```python
from build123d import *

# Parameters (mm, degrees)
SKETCH1_W           = 30.5
SKETCH1_H           = 34
BOSS_EXTRUDE1_DEPTH = 1.5
BOSS_EXTRUDE2_DEPTH = 3
SKETCH3_W           = 3
SKETCH3_H           = 8
SKETCH3_W_2         = 8
SKETCH3_H_2         = 3
BOSS_EXTRUDE3_DEPTH = 3
CUT_EXTRUDE1_DEPTH  = 4.0000001
CUT_EXTRUDE2_DEPTH  = 4.0000001
SKETCH6_W           = 8
SKETCH6_H           = 3
CUT_EXTRUDE3_DEPTH  = 4.0000001
CUT_EXTRUDE4_DEPTH  = 4.0000001
CUT_EXTRUDE6_DEPTH  = 4.0000001
SKETCH9_W           = 3
SKETCH9_H           = 4
BOSS_EXTRUDE4_DEPTH = 3
CUT_EXTRUDE7_DEPTH  = 4
FILLET1_R           = 3
BOSS_EXTRUDE5_DEPTH = 3


with BuildPart() as part:
    # Sketch1 → Boss-Extrude1 (new body, symmetric)
    with BuildSketch(Plane(origin=(0, 0, 0), x_dir=(1, 0, 0), z_dir=(0, 1, 0))):
        Rectangle(SKETCH1_W, SKETCH1_H)
    extrude(amount=BOSS_EXTRUDE1_DEPTH, both=True)

    # Sketch2 → Boss-Extrude2 (add)
    with BuildSketch(Plane(origin=(0, 1.5, 0), x_dir=(1, 0, 0), z_dir=(0, 1, 0))):
        with BuildLine():
            Line((-15.25, 17), (-24.07, 1.308996208))
            add(Edge.make_bspline(
                [(-24.07, 1.308996208), (-25.612124036, -1.43448158), (-30.226003395, -1.5229993), (-46.69780929, -11.088418218), (-55.382760657, -10.307171359), (-55.382760657, -17)],
                knots=[0, 0, 0, 0, 0.221130071, 0.603599568, 1, 1, 1, 1], degree=3))
            Line((-55.382760657, -17), (-15.25, -17))
            Line((-15.25, -17), (-15.25, 17))
        make_face()
    extrude(amount=-BOSS_EXTRUDE2_DEPTH)

    # Sketch3 → Boss-Extrude3 (add)
    with BuildSketch(Plane(origin=(0, 1.5, 0), x_dir=(1, 0, 0), z_dir=(0, 1, 0))):
        with Locations((16.75, 10)):
            Rectangle(SKETCH3_W, SKETCH3_H)
        with Locations((16.75, -10)):
            Rectangle(SKETCH3_W, SKETCH3_H)
        with Locations((-11.25, 18.5)):
            Rectangle(SKETCH3_W_2, SKETCH3_H_2)
        with Locations((11.25, 18.5)):
            Rectangle(SKETCH3_W_2, SKETCH3_H_2)
        with Locations((-51.382760657, -18.5)):
            Rectangle(SKETCH3_W_2, SKETCH3_H_2)
        with Locations((11.25, -18.5)):
            Rectangle(SKETCH3_W_2, SKETCH3_H_2)
        with Locations((-20.066380328, -18.5)):
            Rectangle(SKETCH3_W_2, SKETCH3_H_2)
    extrude(amount=-BOSS_EXTRUDE3_DEPTH)

    # Sketch4 → Cut-Extrude1 (cut, through all)
    with BuildSketch(Plane(origin=(0, 1.5, 0), x_dir=(1, 0, 0), z_dir=(0, 1, 0))):
        Polygon((-2.008190164, -14), (-2.008190164, -12.2), (-3.258190164, -12.2), (-3.258190164, -10), (-5.558190164, -10), (-5.558190164, -12.2), (-6.808190164, -12.2), (-6.808190164, -14), (-5.558190164, -14), (-5.558190164, -17), (-3.258190164, -17), (-3.258190164, -14), align=None)
        Polygon((-33.324570493, -14), (-33.324570493, -12.2), (-34.574570493, -12.2), (-34.574570493, -10), (-36.874570493, -10), (-36.874570493, -12.2), (-38.124570493, -12.2), (-38.124570493, -14), (-36.874570493, -14), (-36.874570493, -17), (-34.574570493, -17), (-34.574570493, -14), align=None)
    extrude(amount=-CUT_EXTRUDE1_DEPTH, mode=Mode.SUBTRACT)

    # Sketch5 → Cut-Extrude2 (cut, through all)
    with BuildSketch(Plane(origin=(0, 1.5, 0), x_dir=(1, 0, 0), z_dir=(0, 1, 0))):
        with BuildLine():
            Line((10.75, 20), (10.75, 7.75))
            ThreePointArc((10.75, 7.75), (2.5, -0.5), (-5.75, 7.75))
            Line((-5.75, 7.75), (-5.75, 20))
            Line((-5.75, 20), (10.75, 20))
        make_face()
    extrude(amount=-CUT_EXTRUDE2_DEPTH, mode=Mode.SUBTRACT)

    # Sketch6 → Cut-Extrude3 (cut, through all)
    with BuildSketch(Plane(origin=(0, 1.5, 0), x_dir=(1, 0, 0), z_dir=(0, 1, 0))):
        with Locations((-11.25, 18.5)):
            Rectangle(SKETCH6_W, SKETCH6_H)
    extrude(amount=-CUT_EXTRUDE3_DEPTH, mode=Mode.SUBTRACT)

    # Sketch7 → Cut-Extrude4 (cut, through all)
    with BuildSketch(Plane(origin=(0, 1.5, 0), x_dir=(1, 0, 0), z_dir=(0, 1, 0))):
        Polygon((-11.65, 17), (-9.35, 17), (-9.35, 14), (-8.1, 14), (-8.1, 12.2), (-9.35, 12.2), (-9.35, 10), (-11.65, 10), (-11.65, 12.2), (-12.9, 12.2), (-12.9, 14), (-11.65, 14), align=None)
    extrude(amount=-CUT_EXTRUDE4_DEPTH, mode=Mode.SUBTRACT)

    # Sketch8 → Cut-Extrude6 (cut, through all)
    with BuildSketch(Plane(origin=(0, 1.5, 0), x_dir=(1, 0, 0), z_dir=(0, 1, 0))):
        with BuildLine():
            Line((-24.066380328, -17), (-24.066380328, 1.315435696))
            Line((-24.066380328, 1.315435696), (-24.07, 1.308996208))
            add(Edge.make_bspline(
                [(-24.07, 1.308996208), (-25.612124036, -1.43448158), (-30.226003395, -1.5229993), (-46.69780929, -11.088418218), (-55.382760657, -10.307171359), (-55.382760657, -17)],
                knots=[0, 0, 0, 0, 0.221130071, 0.603599568, 1, 1, 1, 1], degree=3))
            Line((-55.382760657, -17), (-55.382760657, -20))
            Line((-55.382760657, -20), (-47.382760657, -20))
            Line((-47.382760657, -20), (-47.382760657, -17))
            Line((-47.382760657, -17), (-36.874570493, -17))
            Line((-36.874570493, -17), (-36.874570493, -14))
            Line((-36.874570493, -14), (-38.124570493, -14))
            Line((-38.124570493, -14), (-38.124570493, -12.2))
            Line((-38.124570493, -12.2), (-36.874570493, -12.2))
            Line((-36.874570493, -12.2), (-36.874570493, -10))
            Line((-36.874570493, -10), (-34.574570493, -10))
            Line((-34.574570493, -10), (-34.574570493, -12.2))
            Line((-34.574570493, -12.2), (-33.324570493, -12.2))
            Line((-33.324570493, -12.2), (-33.324570493, -14))
            Line((-33.324570493, -14), (-34.574570493, -14))
            Line((-34.574570493, -14), (-34.574570493, -17))
            Line((-34.574570493, -17), (-24.066380328, -17))
        make_face()
    extrude(amount=-CUT_EXTRUDE6_DEPTH, mode=Mode.SUBTRACT)

    # Sketch9 → Boss-Extrude4 (add)
    with BuildSketch(Plane(origin=(0, 1.5, 0), x_dir=(1, 0, 0), z_dir=(0, 1, 0))):
        with Locations((-25.566380328, -11)):
            Rectangle(SKETCH9_W, SKETCH9_H)
    extrude(amount=-BOSS_EXTRUDE4_DEPTH)

    # Sketch10 → Cut-Extrude7 (cut, through all)
    with BuildSketch(Plane(origin=(0, 1.5, 0), x_dir=(1, 0, 0), z_dir=(0, 1, 0))):
        with BuildLine():
            Line((-21.066380328, 0.530062836), (-21.066380328, -14.173024042))
            Line((-21.066380328, -14.173024042), (-9.808190164, -14.173024042))
            Line((-9.808190164, -14.173024042), (-9.808190164, -7))
            Line((-9.808190164, -7), (0.991809836, -7))
            Line((0.991809836, -7), (0.991809836, -14.173024042))
            Line((0.991809836, -14.173024042), (12.25, -14.173024042))
            Line((12.25, -14.173024042), (12.25, 2.13751392))
            ThreePointArc((12.25, 2.13751392), (-0.04063544, -3.20936456), (-8.72497216, 7))
            Line((-8.72497216, 7), (-17.429592871, 7))
            Line((-17.429592871, 7), (-21.066380328, 0.530062836))
        make_face()
    extrude(amount=-CUT_EXTRUDE7_DEPTH, mode=Mode.SUBTRACT)

    # Fillet1
    fillet1_edges = [part.edges().sort_by_distance(p)[0] for p in [
        (-21.066380328, 0, -0.530062836),
        (-17.429592871, 0, -7),
        (-8.72497216, 0, -7),
        (12.25, 0, -2.13751392),
        (12.25, 0, 14.173024042),
        (0.991809836, 0, 14.173024042),
        (-9.808190164, 0, 7),
        (-9.808190164, 0, 14.173024042),
        (-21.066380328, 0, 14.173024042),
    ]]
    fillet(fillet1_edges, radius=FILLET1_R)

    # Sketch11 → Boss-Extrude5 (add)
    with BuildSketch(Plane(origin=(0, 1.5, 0), x_dir=(1, 0, 0), z_dir=(0, 1, 0))):
        with BuildLine():
            Line((-4.256338517, -7), (0.991809836, -7))
            ThreePointArc((0.991809836, -7), (1.882552513, -4.608606487), (4.120680317, -3.382649968))
            ThreePointArc((4.120680317, -3.382649968), (0.464289311, -3.31428407), (-2.97698799, -2.076754426))
            ThreePointArc((-2.97698799, -2.076754426), (-1.712960608, -5.03307181), (-4.256338517, -7))
        make_face()
    extrude(amount=-BOSS_EXTRUDE5_DEPTH)


solid = part.part
```
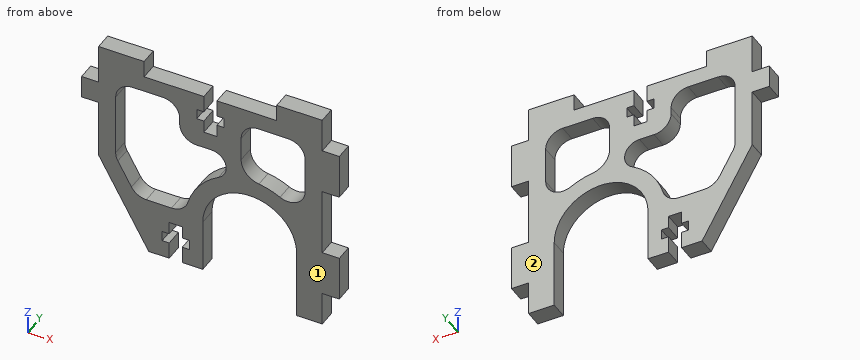
Could you check a few things on this model? Use its own coordinates, in mm. Face numbers are marked on the shaded views. Give positions to 0.01 mm unless a question says otherwise; leave off trailing zeros. Order: outer loops, then holes, each group sorted by start corner. A loop starts at its lowest first (then second) coordinate and runs counter-clockwise, first axis right, second up.
Q1. Suppose I cut it at B-B, the plane x = 2. Write out the boundary of the cut face in (y, z).
Q2. Suppose I cut it at A-A, the plane z = 5.5. Write out the boundary of the cut face in (x, y).
Q3. I'm going to push flat-ended pins straight in: P1, Ø1.5, axis at x = -26.5, y = 0, coming from the -Z side; P2, Ø1.4, axis at x = -6.5, y = -0.5, coming from the +Z side; P3, Ø1, axis at y = 0, z = -4, coming from the -X side. Where does each tip first touch, or does it pass through?
Q4. We'd pull the mould along Y, two halves only. Please class the marked faces 1 and 2: +Y half, -Y half, draft (parallel to the pull), parting line (faces both ways), or undercut.
Q5. If I drill on line 1 along Z through (x, y) = (-14, 0.05); line 2 along X through (y, z) = (0.6, -6.5); line 3 along Z through (x, y) = (-6.5, -0.4), over which ranges is the centre line in solid material (lowest first)?
Q6. Suppose I cut it at D-D, the plane x = 8.5. Write out the boundary of the cut face in (y, z).
Q7. Suppose I cut it at C-C, the plane y = -0.05. Count the separate pieces of the cut face and the enclosed holes in it, and give its area (3 significant figures).
Solution:
1. outline: (-1.5, 0.48) - (1.5, 0.48) - (1.5, 4.48) - (-1.5, 4.48) - close; (-1.5, 13.42) - (1.5, 13.42) - (1.5, 17) - (-1.5, 17) - close
2. outline: (-24.07, -1.5) - (-21.07, -1.5) - (-21.07, 1.5) - (-24.07, 1.5) - close; (-1.88, -1.5) - (1.31, -1.5) - (1.31, 1.5) - (-1.88, 1.5) - close; (12.25, -1.5) - (15.25, -1.5) - (15.25, 1.5) - (12.25, 1.5) - close
3. P1: stops at z = 9
3. P2: stops at z = 17
3. P3: stops at x = -22.84
4. face 1: -Y half
4. face 2: +Y half
5. line 1: z = -17 to -7, 14.17 to 17
5. line 2: x = -21.15 to -17.33, -9.59 to -5.65, 10.65 to 18.25
5. line 3: z = -17 to -1, 7 to 12.2, 14 to 17
6. outline: (-1.5, -2.09) - (1.5, -2.09) - (1.5, 1.9) - (-1.5, 1.9) - close; (-1.5, 14.17) - (1.5, 14.17) - (1.5, 20) - (-1.5, 20) - close
7. separate pieces: 1
7. enclosed holes: 2
7. area: 680 mm2
